The figure shows three views and two pictorial views of one solid part (mm, origin at its lowest corner). Answer the questions. A direction names the side the tool comes from. Coordinates: 2 decimals unless noted, no trailing zeros. Write each loop counter-clockwise with the first axis right and the second up, starting at its lowest first coordinate (ties: lowest second). Pieces come first, ordered by that corner, then holes. Notation, with made-up numbers: M 52.5,8 L 60.5,8 A12 ccw 60.5,30 Z; hole C -31.75,-0.75 d10. An arc over 180 degrees is marked long. Write item = value, one per line.
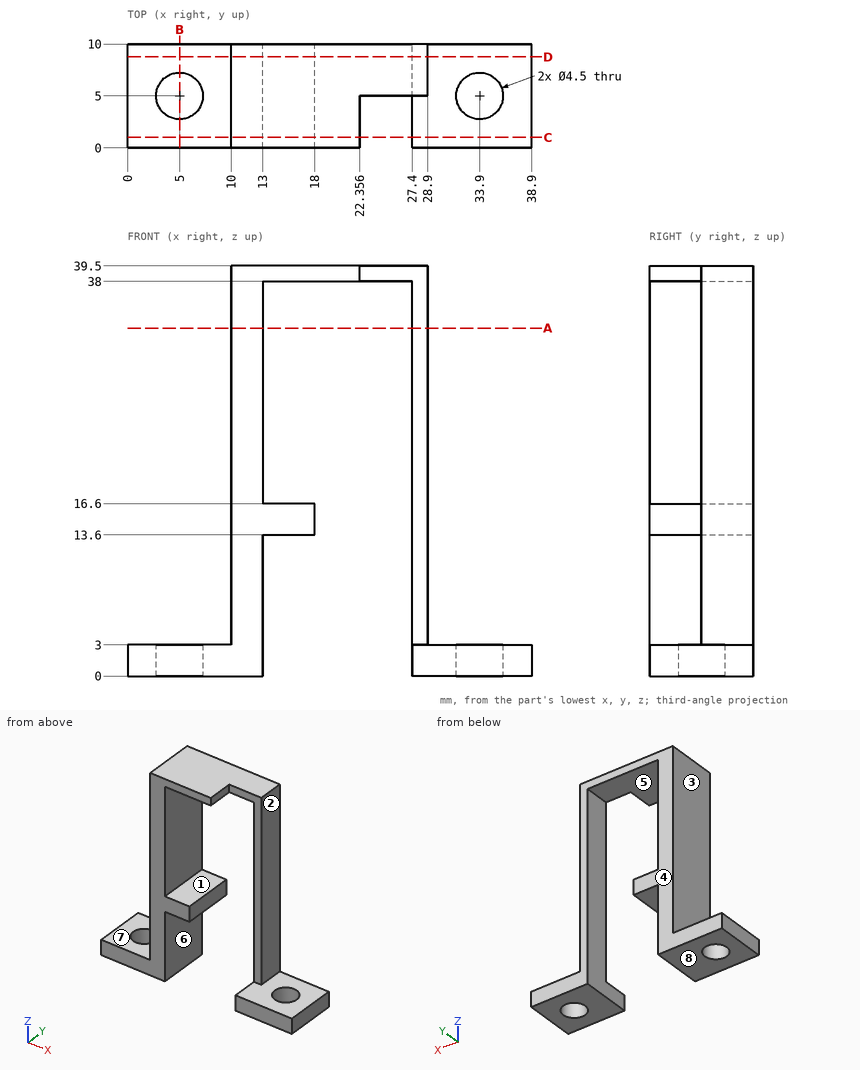
Item 1: Find section B-B (x = 5). Determine the outline of the cut face in (y, z), and give its area (3 significant figures).
Worked answers:
outline = M 0,0 L 2.75,0 L 2.75,3 L 0,3 Z; M 7.25,0 L 10,0 L 10,3 L 7.25,3 Z
area = 16.5 mm²
Item 2: Find section D-D (y = 8.75). Determine the outline of the cut face in (x, z).
Worked answers:
outline = M 0,0 L 13,0 L 13,13.6 L 18,13.6 L 18,16.6 L 13,16.6 L 13,38 L 27.4,38 L 27.4,0 L 38.9,0 L 38.9,3 L 28.9,3 L 28.9,39.5 L 10,39.5 L 10,3 L 0,3 Z
Item 3: Which of the six approach directions +Z, -Z, +X, -X, +Y, -Y give full straight-line access (tool end or side, diameter ignored) to the marked faces 5, 6, 7 and 8?
Worked answers:
face_5 = +Y, -Y
face_6 = -Z, +Y, -Y
face_7 = +Z, -X, +Y, -Y
face_8 = -Z, +X, -X, +Y, -Y
Item 4: Find section C-C (y = 1). Determine the outline of the cut face in (x, z) (1 decimal), and give its area (3 significant figures).
Worked answers:
outline = M 0,0 L 13,0 L 13,13.6 L 18,13.6 L 18,16.6 L 13,16.6 L 13,38 L 22.4,38 L 22.4,39.5 L 10,39.5 L 10,3 L 0,3 Z; M 27.4,0 L 38.9,0 L 38.9,3 L 27.4,3 Z
area = 212 mm²
Item 5: Flat-ended cylindrical pins translate along their axes: pin 1 (4 mm diameter, centred on y = 8, z = 23, fed in from +X); pin 2 (5 mm diameter, centred on x = 16.5, y = 5, fed in from -Z); pin 3 (1.6 mm diameter, centred on y = 2.5, z = 39, fed in from +X); pin 4 (3 mm diameter, centred on x = 5.5, y = 5.5, fed in from -Z). Find the tip coordinate at first contact, or state that the pin passes through.
Worked answers:
pin_1 = 28.9
pin_2 = 13.6
pin_3 = 22.36
pin_4 = through
Item 6: Find section A-A (z = 33.5). Determine the outline of the cut face in (x, y), and give its area (3 significant figures).
Worked answers:
outline = M 10,0 L 13,0 L 13,10 L 10,10 Z; M 27.4,5 L 28.9,5 L 28.9,10 L 27.4,10 Z
area = 37.5 mm²
Item 7: Consider line 1 along X through (y, z) = (9.25, 7.5); line 2 along Z through (x, y) = (14.5, 4); line 3 along Y through (x, z) = (5, 2.15). Determine where each line is inside the solid, lowest interval first. Write a range as from..to.
Worked answers:
line_1 = 10..13, 27.4..28.9
line_2 = 13.6..16.6, 38..39.5
line_3 = 0..2.75, 7.25..10
Item 8: For a pull along X with two mould halves and no side action, classify the marked faces 1, 2, 3 and 4 as released by +X, released by -X, zero draft, split by the parting line, or undercut.
Worked answers:
face_1 = undercut
face_2 = released by +X
face_3 = released by -X
face_4 = zero draft
